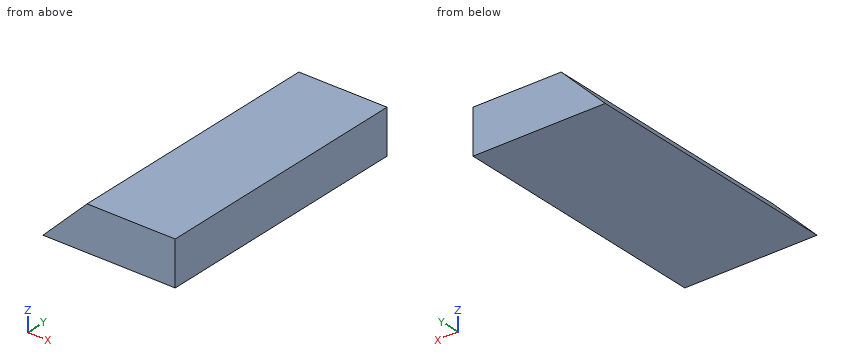
```python
from build123d import *

# Parameters (mm, degrees)
F0_W     = 38.1
F0_H     = 76.2
F1_DEPTH = 12.7
F2_SIZE2 = 12.69999
F2_SIZE  = 12.69999


# Not quite as in the source:
# - a fillet or chamfer is up to 0.001 mm smaller than in the source, because OpenCascade refuses the exact size


with BuildPart() as f1:
    # F0 (on Top) → F1 (new body)
    with BuildSketch(Plane.XY):
        with Locations((4.4191572815, 4.9848316369)):
            Rectangle(F0_W, F0_H)
    extrude(amount=F1_DEPTH)

    # F2 (size 12.7 and 12.7 in the source; OpenCascade refuses exactly that, so slightly less here)
    f2_edges = [f1.edges().sort_by_distance(p)[0] for p in [
        (-14.630843, 4.984832, 12.7),
    ]]
    chamfer(f2_edges, length=F2_SIZE, length2=F2_SIZE2)


solid = f1.part
```
CAD build for the part. Positions are in the model's coordinates, mm. Coordinates: 2 decimals unless noted, no trailing zeros. Write each loop counter-clockwise with the first axis right and the second up, starting at its lowest first coordinate (ties: lowest second). Pieces come first, ordered by that corner, then holes.
(1) Cut at B-B, the plane x = -11. List the corners of the cut face in (y, z).
(2) Drill centre lines: probe 1 along Z at (x, y) = (-5, -27.5); probe 2 along Z at (x, y) = (-13, 13); probe 3 along X at (y, z) = (-7.5, 7.5). Where is each one in solid material? Low to high.
(3) Cut at C-C, the plane z = 3.25. List the corners of the cut face in (x, y), and give its area (3 significant figures).
(4) Flat gauge pin, fed straight in: pin 1 (1.5 mm diameter, centred on y = -10, z = 9.5, fed in from -X). Where does the tip first touch, or does it go through?
Geometry says:
1. outline: (-33.12, 0) - (43.08, 0) - (43.08, 3.63) - (-33.12, 3.63) - close
2. probe 1: z = 0 to 9.63
2. probe 2: z = 0 to 1.63
2. probe 3: x = -7.13 to 23.47
3. outline: (-11.38, -33.12) - (23.47, -33.12) - (23.47, 43.08) - (-11.38, 43.08) - close
3. area: 2,660 mm2
4. pin 1: stops at x = -5.88
